Source: CAD feature listing. Evaluate the final solid. Frame: model axes, mm. Face numbers are marked on the shaded views. A direction names the side the tool comes from. Coordinates: 2 decimals unless noted, no trailing zeros. Loops run counter-clockwise (first coordinate to the right, second up) from the corner with the lowest first, then second, coordinate; pieces in that order, holes last.
Item 1: Line query: probe 1 along X at (y, z) = (2.2, 0); probe 2 along Y at (x, z) = (-5, -3); probe 3 along X at (y, z) = (36.5, 0). Output: solid intervals per line, ascending.
Item 2: Pin query (flat end, axial travel): pin 1 Ø5 at (x, z) = (0, 0.5) entering from -Y; pin 2 Ø7 at (x, z) = (8.5, -1.5) entering from +Y; pin 3 Ø2 at (x, z) = (0, 9) entering from +Y; pin 4 Ø1.5 at (x, z) = (8, 9) entering from +Y. Return the tip coordinate at first contact, or that it passes through.
Item 3: Pull-direction query (Z, two-part tool) for the marked faces 1, 2 and 3; classes: +Z half, -Z half, draft (parallel to the pull), parting line (faces both ways), or undercut.
Item 4: Section query C-C, the plane z = -8.7. Return the cut outline in (x, y), then the cut area to 3 significant figures.
Item 5: Section query A-A, the plane y = 12.5. Return the cut outline in (x, z).
Item 6: Reachability of the marked faces 4, 5 and 6 from +Z, -Z, +X, -X, +Y, -Y: full face, straight path, thin tool, end or side. Return the list, or none.
Item 7: Section query B-B, the plane x = 8.7. Return the cut outline in (y, z).
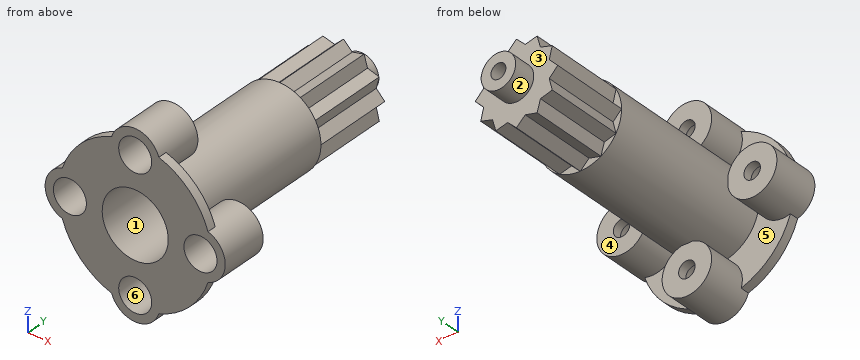
```python
from build123d import *

# Parameters (mm, degrees)
SKETCH1_R            = 10.2
BOSS_EXTRUDE1_DEPTH  = 1.2
SKETCH3_R            = 5.5
BOSS_EXTRUDE2_DEPTH  = 22.8
SKETCH6_R            = 3.3
BOSS_EXTRUDE7_DEPTH  = 6.3
SKETCH7_R            = 2.2
CUT_EXTRUDE1_DEPTH   = 5.1
SKETCH8_R            = 1.1
CUT_EXTRUDE2_DEPTH   = 1.2
CIRPATTERN1_COUNT    = 4
SKETCH9_R            = 4.4
CUT_EXTRUDE3_DEPTH   = 22.8
SKETCH10_R           = 4.5
BOSS_EXTRUDE8_DEPTH  = 10.6
BOSS_EXTRUDE9_DEPTH  = 10.6
CIRPATTERN2_COUNT    = 12
SKETCH12_R           = 3.2
CUT_EXTRUDE4_DEPTH   = 10.6
SKETCH13_R           = 2.3
BOSS_EXTRUDE10_DEPTH = 3
SKETCH14_R           = 1
CUT_EXTRUDE5_DEPTH   = 3
BOSS_EXTRUDE11_DEPTH = 0.1


with BuildPart() as part:
    # Sketch1 → Boss-Extrude1 (new body)
    with BuildSketch(Plane(origin=(0, 0, 0), x_dir=(1, 0, 0), z_dir=(0, 1, 0))):
        with Locations(Location((0, 0, 0), (0, 0, 270))):
            Circle(SKETCH1_R)
    extrude(amount=BOSS_EXTRUDE1_DEPTH)

    # Sketch3 → Boss-Extrude2 (add)
    with BuildSketch(Plane(origin=(0, 1.2, 0), x_dir=(1, 0, 0), z_dir=(0, 1, 0))):
        with Locations(Location((0, 0, 0), (0, 0, 270))):
            Circle(SKETCH3_R)
    extrude(amount=BOSS_EXTRUDE2_DEPTH)

    # Sketch6 → Boss-Extrude7 (add)
    with BuildSketch(Plane.XZ):
        with Locations((8.7, 0)):
            Circle(SKETCH6_R)
    boss_extrude7 = extrude(amount=-BOSS_EXTRUDE7_DEPTH)

    # Sketch7 → Cut-Extrude1 (cut)
    with BuildSketch(Plane.XZ):
        with Locations(Location((8.7, 0, 0), (0, 0, 270))):
            Circle(SKETCH7_R)
    cut_extrude1 = extrude(amount=-CUT_EXTRUDE1_DEPTH, mode=Mode.SUBTRACT)

    # Sketch8 → Cut-Extrude2 (cut)
    with BuildSketch(Plane(origin=(0, 6.3, 0), x_dir=(1, 0, 0), z_dir=(0, 1, 0))):
        with Locations(Location((8.7, 0, 0), (0, 0, 270))):
            Circle(SKETCH8_R)
    cut_extrude2 = extrude(amount=-CUT_EXTRUDE2_DEPTH, mode=Mode.SUBTRACT)

    # CirPattern1: Boss-Extrude7, Cut-Extrude1, Cut-Extrude2 ×4 about axis
    cirpattern1_axis = Axis((0, 0, 0), (0, 1, 0))
    add([boss_extrude7.rotate(cirpattern1_axis, i * 360 / CIRPATTERN1_COUNT) for i in range(1, CIRPATTERN1_COUNT)])
    add([cut_extrude1.rotate(cirpattern1_axis, i * 360 / CIRPATTERN1_COUNT) for i in range(1, CIRPATTERN1_COUNT)], mode=Mode.SUBTRACT)
    add([cut_extrude2.rotate(cirpattern1_axis, i * 360 / CIRPATTERN1_COUNT) for i in range(1, CIRPATTERN1_COUNT)], mode=Mode.SUBTRACT)

    # Sketch9 → Cut-Extrude3 (cut)
    with BuildSketch(Plane(origin=(0, 0, 0), x_dir=(-1, 0, 0), z_dir=(0, -1, 0))):
        with Locations(Location((0, 0, 0), (0, 0, 90))):
            Circle(SKETCH9_R)
    extrude(amount=-CUT_EXTRUDE3_DEPTH, mode=Mode.SUBTRACT)

    # Sketch10 → Boss-Extrude8 (add)
    with BuildSketch(Plane(origin=(0, 24, 0), x_dir=(1, 0, 0), z_dir=(0, 1, 0))):
        with Locations(Location((0, 0, 0), (0, 0, 270))):
            Circle(SKETCH10_R)
    extrude(amount=BOSS_EXTRUDE8_DEPTH)

    # Sketch11 → Boss-Extrude9 (add)
    with BuildSketch(Plane(origin=(0, 24, 0), x_dir=(1, 0, 0), z_dir=(0, 1, 0))):
        Polygon((-1.2, 4.337049688), (1.2, 4.337049688), (0, 5.5), align=None)
    boss_extrude9 = extrude(amount=BOSS_EXTRUDE9_DEPTH)

    # CirPattern2: Boss-Extrude9 ×12 about axis
    cirpattern2_axis = Axis((0, 0, 0), (0, 1, 0))
    for i in range(1, CIRPATTERN2_COUNT):
        add(boss_extrude9.rotate(cirpattern2_axis, i * 360 / CIRPATTERN2_COUNT))

    # Sketch12 → Cut-Extrude4 (cut)
    with BuildSketch(Plane.XZ.offset(-22.8)):
        with Locations(Location((0, 0, 0), (0, 0, 270))):
            Circle(SKETCH12_R)
    extrude(amount=-CUT_EXTRUDE4_DEPTH, mode=Mode.SUBTRACT)

    # Sketch13 → Boss-Extrude10 (add)
    with BuildSketch(Plane(origin=(0, 34.6, 0), x_dir=(1, 0, 0), z_dir=(0, 1, 0))):
        with Locations(Location((0, 0, 0), (0, 0, 270))):
            Circle(SKETCH13_R)
    extrude(amount=BOSS_EXTRUDE10_DEPTH)

    # Sketch14 → Cut-Extrude5 (cut)
    with BuildSketch(Plane(origin=(0, 37.6, 0), x_dir=(1, 0, 0), z_dir=(0, 1, 0))):
        with Locations(Location((0, 0, 0), (0, 0, 270))):
            Circle(SKETCH14_R)
    extrude(amount=-CUT_EXTRUDE5_DEPTH, mode=Mode.SUBTRACT)

    # Sketch15 → Boss-Extrude11 (add)
    with BuildSketch(Plane(origin=(0, 1.2, 0), x_dir=(1, 0, 0), z_dir=(0, 1, 0))):
        Polygon((-5.03433242, -3.66566758), (-3.596315227, -5.103684773), (-3.748047753, -5.2554173), (-5.186064947, -3.817400106), align=None)
    extrude(amount=BOSS_EXTRUDE11_DEPTH)


solid = part.part
```
Verdict:
1. probe 1: x = -12 to -10.9, -6.5 to -4.4, 4.4 to 6.5, 10.9 to 12
1. probe 2: y = 0 to 1.2
1. probe 3: x = -2.3 to -1, 1 to 2.3
2. pin 1: stops at y = 33.4
2. pin 2: stops at y = 34.6
2. pin 3: stops at y = 6.3
2. pin 4: passes through
3. face 1: undercut
3. face 2: parting line
3. face 3: draft
4. outline: (-5.32, 0) - (-2.2, 0) - (-2.2, 5.1) - (-1.1, 5.1) - (-1.1, 6.3) - (-3.3, 6.3) - (-3.3, 1.2) - (-5.32, 1.2) - close; (1.1, 5.1) - (2.2, 5.1) - (2.2, 0) - (5.32, 0) - (5.32, 1.2) - (3.3, 1.2) - (3.3, 6.3) - (1.1, 6.3) - close
4. area: 21.4 mm2
5. outline: circle Ø11 at (0, 0); hole circle Ø8.8 at (0, 0)
6. face 4: +Z, -Z, +X, +Y
6. face 5: +Y
6. face 6: -Y
7. outline: (0, -5.32) - (1.2, -5.32) - (1.2, -3.3) - (6.3, -3.3) - (6.3, -1.1) - (5.1, -1.1) - (5.1, -2.2) - (0, -2.2) - close; (0, 2.2) - (5.1, 2.2) - (5.1, 1.1) - (6.3, 1.1) - (6.3, 3.3) - (1.2, 3.3) - (1.2, 5.32) - (0, 5.32) - close
